Input: part model. Units: mm. Frame: model coordinates. Coordinates: 2 decimals unless noted, no trailing zeros. Write each loop counter-clockwise with the first axis right and the second up, starting at its lowest first coordinate (ties: lowest second). Pieces come first, ordered by that corner, then holes. Notation, with made-up numbers: (-21, -24.5) - (28, -24.5) arc R25 cw to (28, 0.5) - close; hole circle Ø5 at (72.5, 11). An arc over 180 degrees is marked (long way). Use CSV: the item, a comma, the result in double quotes.
```python
from build123d import *

# Parameters (mm, degrees)
CROQUIS1_W              = 190
CROQUIS1_H              = 190
SALIENTE_EXTRUIR1_DEPTH = 2
CROQUIS2_R              = 4
CORTAR_EXTRUIR2_DEPTH   = 4


with BuildPart() as part:
    # Croquis1 → Saliente-Extruir1 (new, symmetric)
    with BuildSketch(Plane.XY):
        with Locations((95, 95)):
            Rectangle(CROQUIS1_W, CROQUIS1_H)
    extrude(amount=SALIENTE_EXTRUIR1_DEPTH, both=True)

    # Croquis2 → Cortar-Extruir2 (cut)
    with BuildSketch(Plane.XY.offset(2)):
        with Locations((95, 168.86)):
            Circle(CROQUIS2_R)
        with Locations((158.938655561, 131.945)):
            Circle(CROQUIS2_R)
        with Locations((158.938655561, 58.115)):
            Circle(CROQUIS2_R)
        with Locations((95, 21.2)):
            Circle(CROQUIS2_R)
        with Locations((31.061344439, 58.115)):
            Circle(CROQUIS2_R)
        with Locations((31.061344439, 131.945)):
            Circle(CROQUIS2_R)
    extrude(amount=-CORTAR_EXTRUIR2_DEPTH, mode=Mode.SUBTRACT)


solid = part.part
```
(1) Pin query (flat end, axial travel): pin 1 Ø9 at (x, y) = (31.06, 131.94) entering from -Z. Return the tip coordinate at first contact, or that it passes through.
Check values:
pin 1,"z = -2"
(2) Ray query, probe 1 along Y at (x, z) = (95, 0.95); probe 2 along Y at (x, z) = (93.5, 1.05); probe 3 along X at (y, z) = (134, 1.6). Return the intervals inside material, ascending. Write a range as from..to.
Check values:
probe 1,"0..17.2, 25.2..164.86, 172.86..190"
probe 2,"0..17.49, 24.91..165.15, 172.57..190"
probe 3,"0..27.63, 34.49..155.51, 162.37..190"
(3) Draft query along X for faces 1 (the flat face through (94, 96, -2)), 2 (the cylindrical face through (33.21, 135.32, 0.03)). Return one class per face: pulls with the +X half, pulls with the -X half, needs draft (parallel to the pull), parting line crosses it, or undercut.
Check values:
face 1,"needs draft"
face 2,"undercut"
(4) Cut plane A-A on y = 21.2. Return loops of the section in (x, z).
Check values:
outline,"(0, -2) - (91, -2) - (91, 2) - (0, 2) - close; (99, -2) - (190, -2) - (190, 2) - (99, 2) - close"
(5) Cut plane B-B on x = 95. Return loops of the section in (y, z).
Check values:
outline,"(0, -2) - (17.2, -2) - (17.2, 2) - (0, 2) - close; (25.2, -2) - (164.86, -2) - (164.86, 2) - (25.2, 2) - close; (172.86, -2) - (190, -2) - (190, 2) - (172.86, 2) - close"
